Geometry check sheet. Reference: the model listing, model coordinates, mm. A direction names the side the tool comes from. Coordinates: 2 decimals unless noted, no trailing zeros. Loops run counter-clockwise (first coordinate to the right, second up) from the corner with the lowest first, then second, coordinate; pieces in that order, holes last. Notation, with made-up numbers: M -21,60 L 27,60 A9 ccw 27,70 Z; hole C -2,75.5 d10. An arc over 180 degrees is marked long. Use CSV: the item, a comma, the result in double quotes.
```python
from build123d import *

# Parameters (mm, degrees)
CROQUIS1_W                   = 70
CROQUIS1_H                   = 100
SALIENTE_EXTRUIR2_DEPTH      = 5
CROQUIS2_W                   = 5
CROQUIS2_H                   = 100
SALIENTE_EXTRUIR3_DEPTH      = 50
CROQUIS3_W                   = 65
CROQUIS3_H                   = 5
SALIENTE_EXTRUIR4_DEPTH      = 45
CROQUIS4_W                   = 65
CROQUIS4_H                   = 5
SALIENTE_EXTRUIR5_DEPTH      = 45
CROQUIS5_W                   = 5
CROQUIS5_H                   = 100
SALIENTE_EXTRUIR6_DEPTH      = 30
REDONDEO2_R                  = 10
REDONDEO3_R                  = 10
REDONDEO4_R                  = 10
REDONDEO5_R                  = 10
SALIENTE_EXTRUIR8_DEPTH      = 2.5
SALIENTE_EXTRUIR8_DEPTH_BACK = 2.5
CROQUIS10_W                  = 65
CROQUIS10_H                  = 20
SALIENTE_EXTRUIR9_DEPTH      = 37
CROQUIS12_W                  = 5
CROQUIS12_H                  = 100
SALIENTE_EXTRUIR10_DEPTH     = 30
REDONDEO10_R                 = 10
REDONDEO11_R                 = 10
REDONDEO13_R                 = 10
REDONDEO16_R                 = 10


with BuildPart() as part:
    # Croquis1 → Saliente-Extruir2 (new body)
    with BuildSketch(Plane(origin=(0, 0, 0), x_dir=(1, 0, 0), z_dir=(0, 1, 0))):
        Rectangle(CROQUIS1_W, CROQUIS1_H)
    extrude(amount=SALIENTE_EXTRUIR2_DEPTH)

    # Croquis2 → Saliente-Extruir3 (add)
    with BuildSketch(Plane(origin=(0, 5, 0), x_dir=(1, 0, 0), z_dir=(0, 1, 0))):
        with Locations((-32.5, 0)):
            Rectangle(CROQUIS2_W, CROQUIS2_H)
    extrude(amount=SALIENTE_EXTRUIR3_DEPTH)

    # Croquis3 → Saliente-Extruir4 (add)
    with BuildSketch(Plane(origin=(0, 5, 0), x_dir=(1, 0, 0), z_dir=(0, 1, 0))):
        with Locations((2.5, -47.5)):
            Rectangle(CROQUIS3_W, CROQUIS3_H)
    extrude(amount=SALIENTE_EXTRUIR4_DEPTH)

    # Croquis4 → Saliente-Extruir5 (add)
    with BuildSketch(Plane(origin=(0, 5, 0), x_dir=(1, 0, 0), z_dir=(0, 1, 0))):
        with Locations((2.5, 47.5)):
            Rectangle(CROQUIS4_W, CROQUIS4_H)
    extrude(amount=SALIENTE_EXTRUIR5_DEPTH)

    # Croquis5 → Saliente-Extruir6 (add)
    with BuildSketch(Plane.XZ):
        with Locations((37.5, 0)):
            Rectangle(CROQUIS5_W, CROQUIS5_H)
    extrude(amount=-SALIENTE_EXTRUIR6_DEPTH)

    # Redondeo2
    redondeo2_edges = [part.edges().sort_by_distance(p)[0] for p in [
        (35, 50, 47.5),
    ]]
    fillet(redondeo2_edges, radius=REDONDEO2_R)

    # Redondeo3
    redondeo3_edges = [part.edges().sort_by_distance(p)[0] for p in [
        (35, 50, -47.5),
    ]]
    fillet(redondeo3_edges, radius=REDONDEO3_R)

    # Redondeo4
    redondeo4_edges = [part.edges().sort_by_distance(p)[0] for p in [
        (-32.5, 55, 50),
    ]]
    fillet(redondeo4_edges, radius=REDONDEO4_R)

    # Redondeo5
    redondeo5_edges = [part.edges().sort_by_distance(p)[0] for p in [
        (-32.5, 55, -50),
    ]]
    fillet(redondeo5_edges, radius=REDONDEO5_R)

    # Croquis10 → Saliente-Extruir8 (add, two sides: drawn at the far end of the back side and taken through both)
    with BuildSketch(Plane.XY.offset(-SALIENTE_EXTRUIR8_DEPTH_BACK)):
        with Locations((2.5, 15)):
            Rectangle(CROQUIS10_W, CROQUIS10_H)
    extrude(amount=SALIENTE_EXTRUIR8_DEPTH + SALIENTE_EXTRUIR8_DEPTH_BACK)

    # Croquis11 → Saliente-Extruir9 (add)
    with BuildSketch(Plane(origin=(40, 0, 0), x_dir=(0, 0, -1), z_dir=(1, 0, 0))):
        Polygon((-50, 30), (-45, 30), (-45, 5), (45.044544461, 5), (45, 30), (50, 30), (50, 0), (-50, 0), align=None)
    extrude(amount=SALIENTE_EXTRUIR9_DEPTH)

    # Croquis12 → Saliente-Extruir10 (add)
    with BuildSketch(Plane.XZ):
        with Locations((79.5, 0)):
            Rectangle(CROQUIS12_W, CROQUIS12_H)
    extrude(amount=-SALIENTE_EXTRUIR10_DEPTH)

    # Redondeo10
    redondeo10_edges = [part.edges().sort_by_distance(p)[0] for p in [
        (77, 5, -0.022272231),
    ]]
    fillet(redondeo10_edges, radius=REDONDEO10_R)

    # Redondeo11
    redondeo11_edges = [part.edges().sort_by_distance(p)[0] for p in [
        (82, 15, -50),
    ]]
    fillet(redondeo11_edges, radius=REDONDEO11_R)

    # Redondeo13
    redondeo13_edges = [part.edges().sort_by_distance(p)[0] for p in [
        (82, 15, 50),
    ]]
    fillet(redondeo13_edges, radius=REDONDEO13_R)

    # Redondeo16
    redondeo16_edges = [part.edges().sort_by_distance(p)[0] for p in [
        (35, 5, -23.75),
        (35, 5, 23.75),
    ]]
    fillet(redondeo16_edges, radius=REDONDEO16_R)


solid = part.part
```
1. Gauge pin test, flat ends, axial feed: P1, Ø5.5, axis at y = 36.5, z = 48, coming from the +X side; P2, Ø3, axis at x = 49, z = 19.5, coming from the +Y side; P3, Ø3, axis at x = -6.5, z = 47, coming from the +Y side. Record the tip position at first contact, or that the pin passes through.
The answers:
P1,"x = 35"
P2,"y = 5"
P3,"y = 50"
2. Section check A-A, the plane y = 34. Record the cut outline in (x, z), plus the area to 3 significant figures.
The answers:
outline,"M -35,-50 L 35,-50 L 35,-45 L -30,-45 L -30,45 L 35,45 L 35,50 L -35,50 Z"
area,"1,150 mm^2"
3. Release check for a two-part mould opening along Z. For faces 1 (the cylindrical face through (-7.818, 49.326, -49.016)), 2 (the flat face through (18, 22, 50)), 3 (the flat face through (-30, 30, 1)), 4 (the flat face through (-3, 50, -47)) record: +Z half, -Z half, draft (parallel to the pull), parting line (faces both ways), or undercut.
The answers:
face 1,"-Z half"
face 2,"+Z half"
face 3,"undercut"
face 4,"draft"
4. Section check B-B, the plane x = 42.5. Record the cut outline in (y, z).
The answers:
outline,"M 0,-50 L 30,-50 L 30,-45 L 5,-45.04 L 5,45 L 30,45 L 30,50 L 0,50 Z"
5. Section check D-D, the plane y = 17. Record the cut outline in (x, z), plus the area to 3 significant figures.
The answers:
outline,"M -35,-50 L 72,-50 A10 ccw 82,-40 L 82,40 A10 ccw 72,50 L -35,50 Z; hole M -30,-45 L 35,-45 L 35,-2.5 L -30,-2.5 Z; hole M -30,2.5 L 35,2.5 L 35,45 L -30,45 Z; hole M 40,-45.02 L 77,-45.02 L 77,45 L 40,45 Z"
area,"2,800 mm^2"
6. Thickness scan on line 1 (Z direction, x = 23.5, y = 8); line 2 (X direction, y = 18.5, z = 40.5); line 3 (Z direction, x = 56.5, y = 28). Record the ranges inside material, lowest first. Write a range as [from, to].
The answers:
line 1,"[-50, -45], [-2.5, 2.5], [45, 50]"
line 2,"[-35, -30], [35, 40], [77, 81.99]"
line 3,"[-50, -45], [45, 50]"
7. Section check C-C, the plane z = 26.5. Record the cut outline in (x, y), plus the area to 3 significant figures.
The answers:
outline,"M -35,0 L 82,0 L 82,30 L 77,30 L 77,15 A10 cw 67,5 L 40,5 L 40,30 L 35,30 L 35,15 A10 cw 25,5 L -30,5 L -30,55 L -35,55 Z"
area,"1,130 mm^2"
8. Set-up check for faces 5 (the flat face through (2, 15, -2.5)), 6 (the flat face through (35, 35, 48)), 7 (the cylindrical face through (78.99, 15.21, -47.15)): record each of +Z, -Z, +X, -X, +Y, -Y from which the full face is reachable in a straight line by a thin tool's end or side.
The answers:
face 5,"+Y"
face 6,"+Z, -Z, +X, +Y"
face 7,"-Z, +X, +Y, -Y"
